Design review of the part built by this model. Coordinates are the model's own, in mm. A direction names the side the tool comes from. Give positions to 0.01 mm unless a question says otherwise; leave off trailing zeros. Order: outer loops, then holes, each group sorted by start corner. A loop starts at its lowest first (then second) coordinate and runs counter-clockwise, first axis right, second up. Notation, with made-up numbers: (38, 36.25) -> (46, 36.25) arc R24 ccw to (46, 66.25) -> close; hole circle Ø7 at (89.5, 89). An arc over 180 degrees is marked (long way). One line per item, written item: value.
from build123d import *

# Parameters (mm, degrees)
SKETCH_1_W          = 36
SKETCH_1_H          = 16
EXTRUDE_1_DEPTH     = 3
SKETCH_2_W          = 20
SKETCH_2_H          = 13
EXTRUDE_2_DEPTH     = 3
SKETCH_3_W          = 20
SKETCH_3_H          = 13
EXTRUDE_3_DEPTH     = 20
FILLET_1_R          = 2
FILLET_2_R          = 1
SKETCH_4_R          = 1.5
CUT_EXTRUDE_1_DEPTH = 46.617978912


with BuildPart() as part:
    # 草图1 → 凸台-拉伸1 (new body)
    with BuildSketch(Plane(origin=(0, 0, 0), x_dir=(0, 0, -1), z_dir=(1, 0, 0))):
        with Locations((18, 8)):
            Rectangle(SKETCH_1_W, SKETCH_1_H)
    extrude(amount=EXTRUDE_1_DEPTH)

    # 草图2 → 凸台-拉伸2 (add)
    with BuildSketch(Plane.ZY):
        with Locations((-18, 8)):
            Rectangle(SKETCH_2_W, SKETCH_2_H)
    extrude(amount=EXTRUDE_2_DEPTH)

    # 草图3 → 凸台-拉伸3 (add)
    with BuildSketch(Plane(origin=(3, 0, 0), x_dir=(0, 0, -1), z_dir=(1, 0, 0))):
        with Locations((18, 8)):
            Rectangle(SKETCH_3_W, SKETCH_3_H)
    extrude(amount=EXTRUDE_3_DEPTH)

    # 圆角1
    fillet_1_edges = [part.edges().sort_by_distance(p)[0] for p in [
        (1.5, 16, 0),
        (1.5, 16, -36),
        (1.5, 0, -36),
        (1.5, 0, 0),
    ]]
    fillet(fillet_1_edges, radius=FILLET_1_R)

    # 圆角2
    fillet_2_edges = [part.edges().sort_by_distance(p)[0] for p in [
        (-1.5, 14.5, -28),
        (-1.5, 1.5, -28),
        (-1.5, 1.5, -8),
        (-1.5, 14.5, -8),
    ]]
    fillet(fillet_2_edges, radius=FILLET_2_R)

    # 草图4 → 切除-拉伸1 (cut, through all)
    with BuildSketch(Plane.ZY):
        with Locations((-31.5, 8)):
            Circle(SKETCH_4_R)
        with Locations((-4.5, 8)):
            Circle(SKETCH_4_R)
    extrude(amount=-CUT_EXTRUDE_1_DEPTH, mode=Mode.SUBTRACT)


solid = part.part
Item 1: Add section A-A on y = 8. Give the boundary of the cut face in (x, z).
Returned:
outline: (-3, -28) -> (0, -28) -> (0, -30) -> (3, -30) -> (3, -28) -> (23, -28) -> (23, -8) -> (3, -8) -> (3, -6) -> (0, -6) -> (0, -8) -> (-3, -8) -> close; (0, -36) -> (3, -36) -> (3, -33) -> (0, -33) -> close; (0, -3) -> (3, -3) -> (3, 0) -> (0, 0) -> close
Item 2: Add section B-B on z = -4.5. Give the boundary of the cut face in (x, y).
Returned:
outline: (0, 0) -> (3, 0) -> (3, 6.5) -> (0, 6.5) -> close; (0, 9.5) -> (3, 9.5) -> (3, 16) -> (0, 16) -> close
Item 3: Add section D-D on y = 5.75. Give the boundary of the cut face in (x, z).
Returned:
outline: (-3, -28) -> (0, -28) -> (0, -36) -> (3, -36) -> (3, -28) -> (23, -28) -> (23, -8) -> (3, -8) -> (3, 0) -> (0, 0) -> (0, -8) -> (-3, -8) -> close
Item 4: Add section C-C on z = -19.5. Give the boundary of the cut face in (x, y), plus the area to 3 significant figures.
Returned:
outline: (-3, 1.5) -> (0, 1.5) -> (0, 0) -> (3, 0) -> (3, 1.5) -> (23, 1.5) -> (23, 14.5) -> (3, 14.5) -> (3, 16) -> (0, 16) -> (0, 14.5) -> (-3, 14.5) -> close
area: 347 mm²
Item 5: Machinability: for faces 1 (the flat face through (-1, 1.5, -18)), 2 (the flat face through (13, 1.5, -18)), 3 (the cylindrical face through (-1.521, 14.215, -8.301)), which of the approach directions +Z, -Z, +X, -X, +Y, -Y give a long, thin tool a straight path to every point of the face, cutting with its end or side? Answer none if there is none.
Returned:
face 1: +Z, -Z, -X, -Y
face 2: +Z, -Z, +X, -Y
face 3: +Z, -X, +Y
Item 6: Clearance check with flat-ended pins moving along their axes: P1, Ø4, axis at y = 13, z = -4.5, coming from the +X side; P2, Ø6.5, axis at x = 17, y = 10.5, coming from the +Z side; P3, Ø6.5, axis at x = 9, y = 7.5, coming from the -Z side. State where each tip first meets the part, or that it passes through.
Returned:
P1: x = 3
P2: z = -8
P3: z = -28
Item 7: To check wall thickness, follow line 1 along Y through (x, z) = (2.25, -4.5); line 2 along Y through (x, z) = (4, -22); line 3 along X through (y, z) = (14.75, -32.5). State the ranges of each line that lie inside material, in increasing order. Write a range as from..to.
Returned:
line 1: 0..6.5, 9.5..16
line 2: 1.5..14.5
line 3: 0..3
